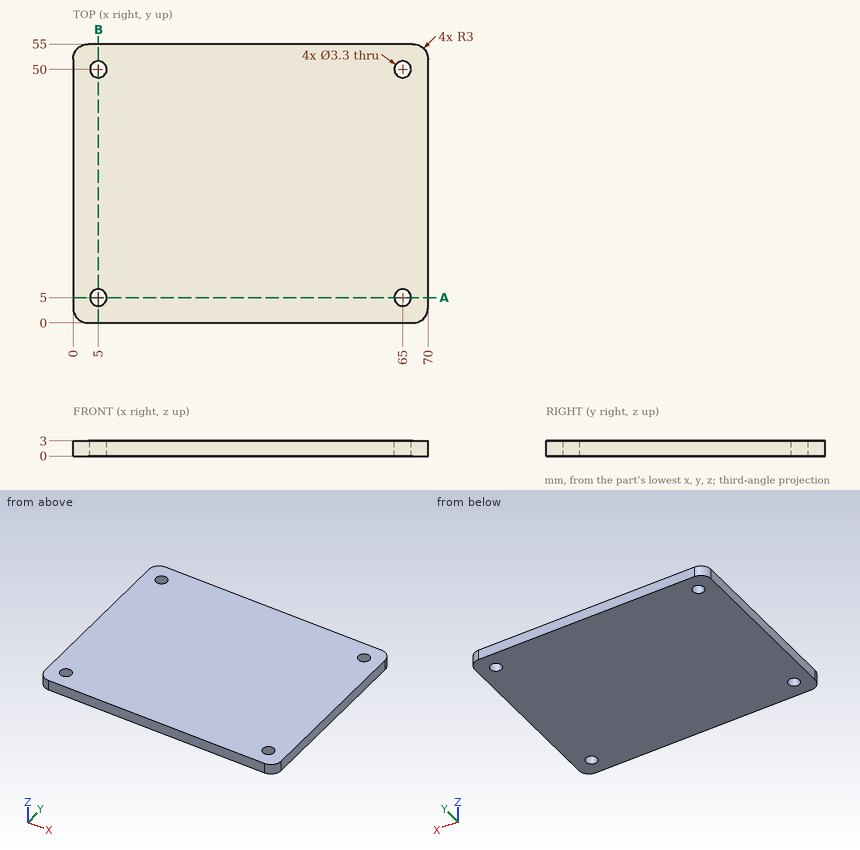
Input: dimensioned drawing with shaded views. Units: mm. Origin: part minimum x, y, z. Round coordinates to 2 decimals unless told otherwise and drop trailing zeros. Loops run counter-clockwise (first coordinate to the right, second up) from the corner with the lowest first, then second, coordinate; pieces in that order, holes last. Notation, with made-up numbers: (40, 36) -> (72, 36) arc R25 ccw to (72, 58) -> close; hole circle Ø6 at (75.25, 17.5). An arc over 180 degrees is marked (long way). Answer as a JSON object with one key per item and string values. Group by question number.
1) Section query A-A on y = 5. Output: boundary loops of the cut face in (x, z).
2) Section query B-B on x = 5. Output: boundary loops of the cut face in (y, z), plus the area to 3 significant figures.
3) Ray query, L1, parallel to X at y = 50, z = 1.05; L2, parallel to Y at x = 5, z = 2.05. Return the intervals inside material, ascending.
4) Pin query (flat end, axial travel): pin 1 (3 mm diameter, centred on x = 5, y = 5, fed in from -Z). Return the tip coordinate at first contact, or that it passes through.
Reply:
{
 "1": {"outline": "(0, 0) -> (3.35, 0) -> (3.35, 3) -> (0, 3) -> close; (6.65, 0) -> (63.35, 0) -> (63.35, 3) -> (6.65, 3) -> close; (66.65, 0) -> (70, 0) -> (70, 3) -> (66.65, 3) -> close"},
 "2": {"outline": "(0, 0) -> (3.35, 0) -> (3.35, 3) -> (0, 3) -> close; (6.65, 0) -> (48.35, 0) -> (48.35, 3) -> (6.65, 3) -> close; (51.65, 0) -> (55, 0) -> (55, 3) -> (51.65, 3) -> close", "area": "145 mm2"},
 "3": {"L1": "x = 0 to 3.35, 6.65 to 63.35, 66.65 to 70", "L2": "y = 0 to 3.35, 6.65 to 48.35, 51.65 to 55"},
 "4": {"pin 1": "passes through"}
}
